Design review of the part built by this model. Coordinates are the model's own, in mm. Face numbers are marked on the shaded views. A direction names the side the tool comes from. Coordinates: 2 decimals unless noted, no trailing zeros. Loops run counter-clockwise (first coordinate to the right, second up) from the corner with the lowest first, then second, coordinate; pieces in that order, holes last. Notation, with made-up numbers: (68, 57.25) -> (125, 57.25) arc R13 cw to (125, 77.25) -> close; hole circle Ø1 at (-8.5, 19). An arc over 180 degrees is marked (long way). One line per item, written item: value. Start each with the question number.
1. Machinability: for the marked faces 5, 6, 7 and 8, which of the approach directions +Z, -Z, +X, -X, +Y, -Y give a long, thin tool a straight path to every point of the face, cutting with its end or side? Answer none if there is none.
2. Insertion check: pin 1 (6 mm diameter, centred on y = 9, z = -15, fed in from -X); pin 2 (4 mm diameter, centred on x = -11.5, y = -1.5, fed in from -Z); pin 3 (1.5 mm diameter, centred on x = -14, y = -15.5, fed in from -Z); pin 4 (12 mm diameter, centred on x = -26.5, z = -3.5, fed in from +Y). Each pin has a flat end and moves straight along its axis. Give the tip position at first contact, or say it passes through.
3. Add section A-A on y = -5.8. Give the number of separate pieces and of enclosed holes in the cut face, plus the area to 3 significant figures.
4. Draft analysis for pull direction Z (two halves, no side actions). For the marked faces 1, 2, 3 and 4, state which applies: pulls with the +Z half, pulls with the -Z half, needs draft (parallel to the pull), parting line crosses it, or undercut.
5. Add section B-B on x = -19. Write out the cut boundary in (y, z), plus the area to 3 significant figures.
6. Add section C-C on z = 0. Write out the cut boundary in (x, y).
7. Add section D-D on x = -15. Write out the cut boundary in (y, z), plus the area to 3 significant figures.
8. For probe 1 along X at (y, z) = (-5.8, 10.3); probe 2 along X at (y, z) = (-24, 1.5); probe 3 along Z at (x, y) = (-22, -4.5), list the stretches that pass through material, from the lowest coordinate up.
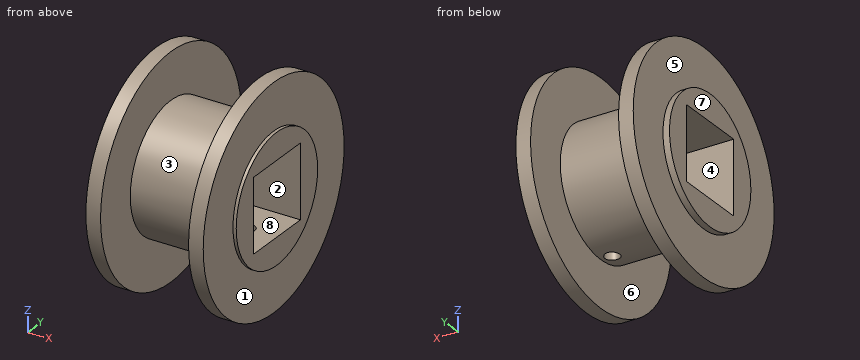
Autodesk Inventor part; units mm, degrees
ref_plane "YZ Plane" through (0, 0, 0) normal (1, 0, 0) x (0, 1, 0)
ref_plane "XZ Plane" through (0, 0, 0) normal (0, 1, 0) x (-1, 0, 0)
ref_plane "XY Plane" through (0, 0, 0) normal (0, 0, 1) x (1, 0, 0)
sketch "Sketch1" plane through (0, 0, 0) normal (0, 0, 1) x (1, 0, 0)
  line L0 (-9, 0) -> (-9, 7.2)
  line L1 (-9, 7.2) -> (-9.6665, 7.2)
  line L2 (-9.6665, 7.2) -> (-9.6665, 16.7)
  line L3 (-9.6665, 16.7) -> (-12.6665, 16.7)
  line L4 (-12.6665, 16.7) -> (-12.6665, 9.4)
  line L5 (-35, 0) -> (-35, 7.2)
  line L6 (-35, 7.2) -> (-33.6665, 7.2)
  line L7 (-33.6665, 7.2) -> (-33.6665, 16.7)
  line L8 (-33.6665, 16.7) -> (-30.6665, 16.7)
  line L9 (-30.6665, 16.7) -> (-30.6665, 7.2)
  line L10 (-41.0656, -5.8) -> (-47.8962, -5.8)
  line L11 (-12.6665, 9.4) -> (-12.6665, 7.2)
  line L12 (-30.6665, 7.2) -> (-12.6665, 7.2)
  line L13 (-35, 0) -> (-35, -5.8)
  line L14 (-9, 0) -> (-9, -5.8)
  line L15 (-9, -5.8) -> (-35, -5.8)
  circle A0 centre (-15, -5.8) radius 1.5
  point P0 (0, 0)
  point P1 (-16.5, -5.8)
  point P2 (-13.5, -5.8)
  dimension "d5" = 3
  dimension "d6" = 45
  dimension "d7" = 26
  dimension "d9" = 3
  dimension "d11" = 18
  dimension "d12" = 26
revolve "Revolution1" add sketch "Sketch1" angle 360 about axis through (-41.0656, -5.8, 0) along (-1, 0, 0) contours L14 L15 A0 L13 L5 L6 L7 L8 L9 L12 L11 L4 L3 L2 L1 L0
sketch "Sketch2" plane through (-9, -5.8, 0) normal (1, 0, 0) x (0, 0, -1)
  line L0 (7.5, -7.5) -> (-7.5, -7.5)
  line L1 (-7.5, -7.5) -> (-7.5, 7.5)
  line L2 (-7.5, 7.5) -> (7.5, 7.5)
  line L3 (7.5, 7.5) -> (7.5, -7.5)
  line L4 (7.5, -7.5) -> (-7.5, 7.5) construction
  line L5 (-7.5, -7.5) -> (7.5, 7.5) construction
  point P0 (0, 5.8)
  point P1 (0, 0)
  dimension "d14" = 15
  dimension "d15" = 15
extrude "Extrusion1" cut sketch "Sketch2" against normal blind 100
extrude "Extrusion2" cut sketch "Sketch1" along normal mid plane 100 contours A0 L15 | L15 A0
Worked answers:
1. face 5: -X
1. face 6: none
1. face 7: +Z, -Z, -X, +Y, -Y
1. face 8: +X, -X
2. pin 1: stops at x = -33.67
2. pin 2: stops at z = -22.38
2. pin 3: stops at z = -9.43
2. pin 4: stops at y = 16.7
3. separate pieces: 4
3. enclosed holes: 0
3. area: 367 mm²
4. face 1: needs draft
4. face 2: undercut
4. face 3: parting line crosses it
4. face 4: undercut
5. outline: circle Ø26 at (-5.8, 0); hole (-13.3, -7.5) -> (1.7, -7.5) -> (1.7, 7.5) -> (-13.3, 7.5) -> close
5. area: 306 mm²
6. outline: (-35, -18.8) -> (-33.67, -18.8) -> (-33.67, -28.3) -> (-30.67, -28.3) -> (-30.67, -18.8) -> (-12.67, -18.8) -> (-12.67, -28.3) -> (-9.67, -28.3) -> (-9.67, -18.8) -> (-9, -18.8) -> (-9, -13.3) -> (-35, -13.3) -> close; (-35, 1.7) -> (-9, 1.7) -> (-9, 7.2) -> (-9.67, 7.2) -> (-9.67, 16.7) -> (-12.67, 16.7) -> (-12.67, 7.2) -> (-30.67, 7.2) -> (-30.67, 16.7) -> (-33.67, 16.7) -> (-33.67, 7.2) -> (-35, 7.2) -> close
7. outline: (-13.3, -7.5) -> (-13.3, 7.5) -> (-7.3, 7.5) -> (-7.3, 12.91) arc R13 ccw to (-7.3, -12.91) -> (-7.3, -7.5) -> close; (-4.3, -12.91) arc R13 ccw to (-4.3, 12.91) -> (-4.3, 7.5) -> (1.7, 7.5) -> (1.7, -7.5) -> (-4.3, -7.5) -> close
7. area: 273 mm²
8. probe 1: x = -35 to -16.5, -13.5 to -9
8. probe 2: x = -33.67 to -30.67, -12.67 to -9.67
8. probe 3: z = -12.93 to -7.5, 7.5 to 12.93
